Source: CAD feature listing. Evaluate the final solid. Frame: model axes, mm. A direction names the side the tool comes from. Round coordinates to 2 decimals unless told otherwise and drop trailing zeros. Write each loop counter-clockwise with the first axis right and the second up, starting at its lowest first coordinate (ties: lowest second). Pieces come first, ordered by that corner, then holes. Notation, with made-up numbers: M -39.5,69.5 L 19.5,69.5 A21 cw 19.5,104.5 Z; hole C -29,33 d4. An arc over 180 degrees is marked long. Answer in a Markdown table with one row per item.
from build123d import *

# Parameters (mm, degrees)
SKETCH_1_R             = 10
SKETCH_1_R_2           = 0.5
SKETCH_1_R_3           = 1.5
EXTRUDE_1_DEPTH        = 2.5
SKETCH_2_R             = 4.5
SKETCH_2_R_2           = 3
EXTRUDE_2_DEPTH        = 2
CUT_EXTRUDE_START      = -1
SKETCH_3_R             = 3
CUT_EXTRUDE_1_DEPTH    = 1
CHAMFER_1_SIZE         = 0.3
HOLE_WIZARD_M3_1_D     = 2.5
HOLE_WIZARD_M3_1_DEPTH = 6.5
HOLE_WIZARD_M3_1_TIP   = 0.751075774


with BuildPart() as part:
    # 草图1 → 凸台-拉伸1 (new body)
    with BuildSketch(Plane.XY):
        Circle(SKETCH_1_R)
        with Locations((0, 7)):
            Circle(SKETCH_1_R_2, mode=Mode.SUBTRACT)
        with Locations((7, 0)):
            Circle(SKETCH_1_R_2, mode=Mode.SUBTRACT)
        with Locations((0, -7)):
            Circle(SKETCH_1_R_2, mode=Mode.SUBTRACT)
        with Locations((-7, 0)):
            Circle(SKETCH_1_R_2, mode=Mode.SUBTRACT)
        Circle(SKETCH_1_R_3, mode=Mode.SUBTRACT)
    extrude(amount=EXTRUDE_1_DEPTH)

    # 草图2 → 凸台-拉伸2 (add)
    with BuildSketch(Plane.XY.offset(2.5)):
        Circle(SKETCH_2_R)
        Circle(SKETCH_2_R_2, mode=Mode.SUBTRACT)
    extrude(amount=EXTRUDE_2_DEPTH)

    # 草图3 → 切除-拉伸1 (cut)
    with BuildSketch(Plane.XY.offset(2.5).offset(CUT_EXTRUDE_START)):
        Circle(SKETCH_3_R)
    extrude(amount=CUT_EXTRUDE_1_DEPTH, mode=Mode.SUBTRACT)

    # 倒角1
    chamfer_1_edges = [part.edges().sort_by_distance(p)[0] for p in [
        (-1.5, 0, 1.5),
    ]]
    chamfer(chamfer_1_edges, length=CHAMFER_1_SIZE)

    # M3 螺纹孔的螺纹孔钻头1
    with Locations(Plane(origin=(0, 0, 0), x_dir=(-1, 0, 0), z_dir=(0, 0, -1))):
        with Locations((0, 7), (7, 0), (0, -7), (-7, 0)):
            Hole(HOLE_WIZARD_M3_1_D / 2, depth=HOLE_WIZARD_M3_1_DEPTH)
            with Locations((0, 0, -(HOLE_WIZARD_M3_1_DEPTH + HOLE_WIZARD_M3_1_TIP / 2))):  # 118° drill point
                Cone(0, HOLE_WIZARD_M3_1_D / 2, HOLE_WIZARD_M3_1_TIP, mode=Mode.SUBTRACT)


solid = part.part
Q1. Material intervals for probe 1 along Y at (x, z) = (0, 0.4); probe 2 along Y at (x, z) = (0, 2.85); probe 3 along X at (y, z) = (-1, 2.45), sorted ascending.
Solutions:
| item | result |
|---|---|
| probe 1 | y = -10 to -8.25, -5.75 to -1.5, 1.5 to 5.75, 8.25 to 10 |
| probe 2 | y = -4.5 to -3, 3 to 4.5 |
| probe 3 | x = -9.95 to -7.75, -6.25 to -2.83, 2.83 to 6.25, 7.75 to 9.95 |
Q2. Pull-direction query (X, two-part tool) for faces 3 (the flat face through (0, -2, 1.5)), 4 (the cylindrical face through (-2.17, -9.76, 1.23)), 5 (the flat face through (0, -2, 0)), 6 (the cylindrical face through (-1.5, 0.07, 0.59)); classes: pulls with the +X half, pulls with the -X half, needs draft (parallel to the pull), parting line crosses it, or undercut.
Solutions:
| item | result |
|---|---|
| face 3 | undercut |
| face 4 | parting line crosses it |
| face 5 | needs draft |
| face 6 | undercut |
Q3. Section B-B (y = 0). Return loops of the section in (x, z).
Solutions:
| item | result |
|---|---|
| outline | M -10,0 L -8.25,0 L -8.25,2.5 L -10,2.5 Z; M -5.75,0 L -1.5,0 L -1.5,1.2 L -1.8,1.5 L -3,1.5 L -3,4.5 L -4.5,4.5 L -4.5,2.5 L -5.75,2.5 Z; M 1.5,0 L 5.75,0 L 5.75,2.5 L 4.5,2.5 L 4.5,4.5 L 3,4.5 L 3,1.5 L 1.8,1.5 L 1.5,1.2 Z; M 8.25,0 L 10,0 L 10,2.5 L 8.25,2.5 Z |
Q4. Contact query for flat-ended pins moving along their axis: pin 1 Ø5 at (x, y) = (0, 0) entering from +Z; pin 2 Ø1.5 at (y, z) = (7, 3) entering from +X. Output: stop coordinate, or through.
Solutions:
| item | result |
|---|---|
| pin 1 | stops at z = 1.5 |
| pin 2 | stops at x = 7.65 |
Q5. Section C-C (z = 1.75). Return loops of the section in (x, y), and give its area (3 significant figures).
Solutions:
| item | result |
|---|---|
| outline | C 0,0 d20; hole C -7,0 d2.5; hole C 0,0 d6; hole C 0,-7 d2.5; hole C 0,7 d2.5; hole C 7,0 d2.5 |
| area | 266 mm2 |
Q6. Access query for faces 1 (the flat face through (1, -3, 4.5)), 2 (the flat face through (4.3, -2.1, 2.5)). Directions: +Z, -Z, +X, -X, +Y, -Y. A direction counts if a zero-diameter tool reaches every point of the face in a straight line with its end or side. Return the directions, or none.
Solutions:
| item | result |
|---|---|
| face 1 | +Z, +X, -X, +Y, -Y |
| face 2 | +Z |
Q7. Section A-A (x = -8). Return loops of the section in (y, z), and give its area (4 significant figures).
Solutions:
| item | result |
|---|---|
| outline | M -6,0 L -0.75,0 L -0.75,2.5 L -6,2.5 Z; M 0.75,0 L 6,0 L 6,2.5 L 0.75,2.5 Z |
| area | 26.25 mm2 |
